from build123d import *

# Parameters (mm, degrees)
SKETCH2_R           = 2.945157041
BOSS_EXTRUDE1_DEPTH = 1
SKETCH3_R           = 3.125
BOSS_EXTRUDE2_DEPTH = 2
FILLET1_R           = 2
FILLET2_R           = 0.5


with BuildPart() as part:
    # Sketch1 → Revolve1 (revolve)
    with BuildSketch(Plane.XY, mode=Mode.PRIVATE) as revolve1_sk:
        with BuildLine():
            Line((2.790292922, 0), (3.125, 0))
            ThreePointArc((3.125, 0), (4.976777415, -4.958274435), (5.60588742, -10.213537089))
            Line((5.60588742, -10.213537089), (5.11812749, -10.213537089))
            ThreePointArc((5.11812749, -10.213537089), (4.52880139, -4.97580968), (2.790292922, 0))
        make_face()
    revolve(revolve1_sk.sketch.rotate(Axis((0, -10.213537089, 0), (0, 1, 0)), 90), axis=Axis((0, -10.213537089, 0), (0, 1, 0)))

    # Sketch2 → Boss-Extrude1 (add)
    with BuildSketch(Plane(origin=(0, 0, 0), x_dir=(1, 0, 0), z_dir=(0, 1, 0))):
        with Locations(Location((0, 0, 0), (0, 0, 270))):
            Circle(SKETCH2_R)
    extrude(amount=BOSS_EXTRUDE1_DEPTH)

    # Sketch3 → Boss-Extrude2 (add)
    with BuildSketch(Plane(origin=(0, 1, 0), x_dir=(1, 0, 0), z_dir=(0, 1, 0))):
        with Locations(Location((0, 0, 0), (0, 0, 270))):
            Circle(SKETCH3_R)
    extrude(amount=BOSS_EXTRUDE2_DEPTH)

    # Fillet1
    # the kernel refuses this fillet: 2 mm, written as the material it adds along each edge
    with BuildSketch(Plane(origin=(0, 0, 0), x_dir=(0, 0, 1), z_dir=(-1, 0, 0))) as fillet1_piece_1:
        with BuildLine():
            CenterArc((4.945157041, 0.828871731), FILLET1_R, 180, 24.483795265)
            Line((3.125, 0), (2.945157041, 0))
            Line((2.945157041, 0), (2.945157041, 0.828871731))
        make_face()
    revolve(axis=Axis((0, 0, 0), (0, 1, 0)))

    # Fillet2
    # the kernel refuses this fillet: 0.5 mm, written as the material it adds along each edge
    with BuildSketch(Plane(origin=(0, 1, 0), x_dir=(0, 0, 1), z_dir=(-1, 0, 0))) as fillet2_piece_1:
        with BuildLine():
            CenterArc((3.458713381, -0.372337723), FILLET2_R, 131.868770298, 55.840101838)
            Line((3.125, 0), (3.091628662, 0.037233772))
            ThreePointArc((3.091628662, 0.037233772), (3.035078521, 0.05), (2.945157041, 0.05))
            Line((2.945157041, 0.05), (2.895157041, 0))
            ThreePointArc((2.895157041, 0), (2.895157041, -0.171128269), (2.913684038, -0.446114522))
            Line((2.913684038, -0.446114522), (2.96323216, -0.43940754))
        make_face()
    revolve(axis=Axis((0, 1, 0), (0, 1, 0)))


solid = part.part
Here's how the part is built. I have some questions about the finished solid (model axes, mm). Round coordinates to 2 decimals unless told otherwise and drop trailing zeros. Return JSON: item names as keys, results as strings. Group by question number.
1. Please list where these lines run through material, in increasing order: probe 1 along Y at (x, z) = (0.25, -1.75); probe 2 along Z at (x, y) = (-2.5, -5.25); probe 3 along Z at (x, y) = (2.5, -2.75).
2. I'm going to push flat-ended pins straight in: pin 1 Ø2 at (y, z) = (-7.5, -1) entering from +X; pin 2 Ø5 at (x, z) = (3, 1.5) entering from -Y; pin 3 Ø4 at (y, z) = (-2.5, 4.5) entering from +X; pin 4 Ø2 at (x, y) = (1, -8) entering from -Z. Where does each tip first touch, or does it pass through?
3. If we mould it in two halves opening along X, with no side actions, what happens to faces 1 (the face through (0.94, 1.99, 2.98)), 2 (the face through (0, 3, 0)), 3 (the face through (0, 0, 0))? For each: pulls with the +X half, pulls with the -X half, needs draft (parallel to the pull), parting line crosses it, or undercut.
Reply:
{
 "1": {"probe 1": "0 to 3", "probe 2": "-4.38 to -3.85, 3.85 to 4.38", "probe 3": "-3.52 to -3, 3 to 3.52"},
 "2": {"pin 1": "x = 5.51", "pin 2": "y = -10.21", "pin 3": "x = 3.64", "pin 4": "z = -5.55"},
 "3": {"face 1": "parting line crosses it", "face 2": "needs draft", "face 3": "undercut"}
}
